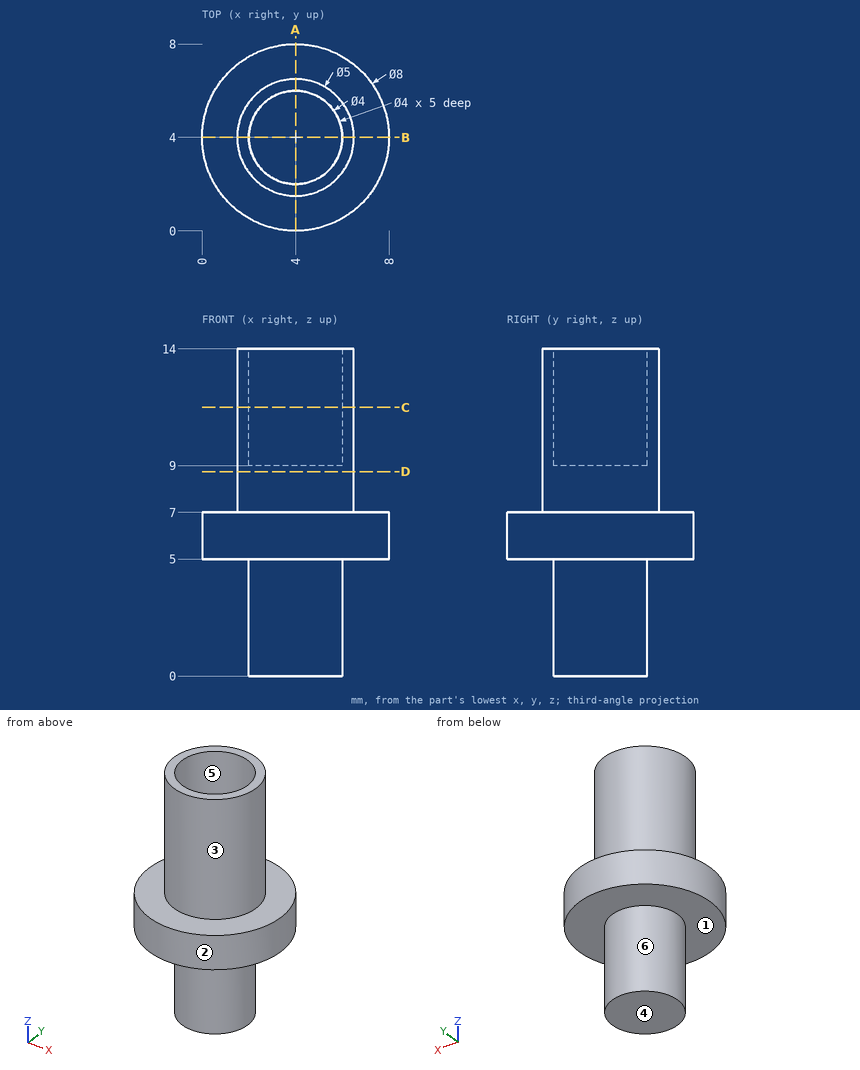
Design review of the part shown in the three views and the two pictorial views. Dimensions are in mm from the part's minimum x, y and z. A direction names the side the tool comes from. Round coordinates to 2 decimals unless told otherwise and drop trailing zeros. Loops run counter-clockwise (first coordinate to the right, second up) from the corner with the lowest first, then second, coordinate; pieces in that order, holes last. Notation, with made-up numbers: (-31.75, 1.25) - (-10.75, 1.25) arc R15 ccw to (-10.75, 30.25) - close; hole circle Ø9 at (70, 54.5). An arc over 180 degrees is marked (long way). One line per item, written item: value. Start each with the question number.
Item 1: The part is to be moulded in two halves that separate along Y. For the marked faces 4, 5 and 6, say which applies: +Y half, -Y half, draft (parallel to the pull), parting line (faces both ways), or undercut.
Item 2: For the marked faces 1, 2 and 3, list the 3-axis set-ups (+Z, -Z, +X, -X, +Y, -Y) from which the entire face can be reached by the end or side of a thin tool; tool diameter is ignored.
Item 3: Take a section at D-D (z = 8.75). Give the boundary of the cut face in (x, y), plus the area to 3 significant figures.
Item 4: Take a section at A-A (x = 4). Give the boundary of the cut face in (y, z).
Item 5: Clearance check with flat-ended pins moving along their axes: pin 1 Ø1.5 at (y, z) = (3.5, 8.5) entering from -X; pin 2 Ø4 at (x, z) = (7, 4) entering from +Y. State where each tip first meets the part, or that it passes through.
Item 6: Take a section at C-C (z = 11.5). Give the boundary of the cut face in (x, y).
Item 7: For L1, parallel to Y at x = 4, z = 10.2; L2, parallel to Z at x = 6.25, y = 5.5; L3, parallel to Z at x = 5.75, y = 4.75, list the stretches that pass through material, from the lowest coordinate up.
Answer below:
1. face 4: draft
1. face 5: undercut
1. face 6: parting line
2. face 1: -Z
2. face 2: +Z, -Z
2. face 3: +Z
3. outline: circle Ø5 at (4, 4)
3. area: 19.6 mm2
4. outline: (0, 5) - (2, 5) - (2, 0) - (6, 0) - (6, 5) - (8, 5) - (8, 7) - (6.5, 7) - (6.5, 14) - (6, 14) - (6, 9) - (2, 9) - (2, 14) - (1.5, 14) - (1.5, 7) - (0, 7) - close
5. pin 1: stops at x = 1.5
5. pin 2: stops at y = 7.79
6. outline: circle Ø5 at (4, 4); hole circle Ø4 at (4, 4)
7. L1: y = 1.5 to 2, 6 to 6.5
7. L2: z = 5 to 7
7. L3: z = 0 to 9
